Geometry: final body of the model. Coordinates: model frame, mm. A direction names the side the tool comes from. Coordinates: 2 decimals unless noted, no trailing zeros. Loops run counter-clockwise (first coordinate to the right, second up) from the corner with the lowest first, then second, coordinate; pieces in that order, holes last. Notation, with made-up numbers: (48.5, 45.25) - (104.5, 45.25) arc R28 cw to (104.5, 65.25) - close; hole circle Ø10 at (-17, -35.5). An arc over 180 degrees is marked (long way). Answer in a Markdown table with one row per item.
from build123d import *

# Parameters (mm, degrees)
SKETCH1_R           = 8.5
BOSS_EXTRUDE1_DEPTH = 61
SKETCH9_R           = 1.7
CUT_EXTRUDE2_DEPTH  = 6.7
SKETCH10_R          = 1
CUT_EXTRUDE3_DEPTH  = 8.7
CIRPATTERN1_COUNT   = 4
SKETCH11_R          = 1.7
CUT_EXTRUDE4_DEPTH  = 8.7


with BuildPart() as part:
    # Sketch1 → Boss-Extrude1 (new body)
    with BuildSketch(Plane.XY):
        with Locations(Location((0, 0, 0), (0, 0, 180))):
            Circle(SKETCH1_R)
    extrude(amount=BOSS_EXTRUDE1_DEPTH)

    # Sketch7 → Cut-Revolve1 (revolve, cut)
    with BuildSketch(Plane(origin=(0, 0, 0), x_dir=(0, 0, -1), z_dir=(1, 0, 0)), mode=Mode.PRIVATE) as cut_revolve1_sk:
        Polygon((-61, 3), (-5, 3), (-1, 1.5), (0, 1.5), (0, 0), (-61, 0), align=None)
    revolve(cut_revolve1_sk.sketch.rotate(Axis((0, 0, 0), (0, 0, 1)), 90), axis=Axis((0, 0, 0), (0, 0, 1)), mode=Mode.SUBTRACT)

    # Sketch9 → Cut-Extrude2 (cut)
    with BuildSketch(Plane(origin=(8.5, 0, 0), x_dir=(0, 0, -1), z_dir=(1, 0, 0))):
        with Locations((-6.641615966, 0)):
            Circle(SKETCH9_R)
    extrude(amount=-CUT_EXTRUDE2_DEPTH, mode=Mode.SUBTRACT)

    # Sketch10 → Cut-Extrude3 (cut)
    with BuildSketch(Plane(origin=(0, 0, 0), x_dir=(0, 0, -1), z_dir=(1, 0, 0))):
        with Locations(Location((-59, 0, 0), (0, 0, 180))):
            Circle(SKETCH10_R)
    cut_extrude3 = extrude(amount=-CUT_EXTRUDE3_DEPTH, mode=Mode.SUBTRACT)

    # CirPattern1: Cut-Extrude3 ×4 about axis
    cirpattern1_axis = Axis((0, 0, 61), (0, 0, 1))
    for i in range(1, CIRPATTERN1_COUNT):
        add(cut_extrude3.rotate(cirpattern1_axis, i * 360 / CIRPATTERN1_COUNT), mode=Mode.SUBTRACT)

    # Sketch11 → Cut-Extrude4 (cut)
    with BuildSketch(Plane(origin=(0, 8.5, 0), x_dir=(1, 0, 0), z_dir=(0, 1, 0))):
        with Locations(Location((0, -31.611405642, 0), (0, 0, 270))):
            Circle(SKETCH11_R)
    extrude(amount=-CUT_EXTRUDE4_DEPTH, mode=Mode.SUBTRACT)


solid = part.part
(1) Ray query, probe 1 along Z at (x, y) = (6.25, 0); probe 2 along Y at (x, z) = (0, 19.5); probe 3 along Z at (x, y) = (0, -4.65). Return the intervals inside material, ascending.
Verdict:
| item | result |
|---|---|
| probe 1 | z = 0 to 4.94, 8.34 to 58, 60 to 61 |
| probe 2 | y = -8.5 to -3, 3 to 8.5 |
| probe 3 | z = 0 to 58, 60 to 61 |
(2) Cut plane D-D on z = 51. Output: boundary loops of the cut face in (x, y), then the cut area to 3 significant figures.
Verdict:
| item | result |
|---|---|
| outline | circle Ø17 at (0, 0); hole circle Ø6 at (0, 0) |
| area | 199 mm² |
(3) Cut plane B-B on z = 59. Output: boundary loops of the cut face in (x, y), then the cut area to 3 significant figures.
Verdict:
| item | result |
|---|---|
| outline | (-8.44, -1) arc R8.5 ccw to (-1, -8.44) - (-1, -2.83) arc R3 cw to (-2.83, -1) - close; (-8.44, 1) - (-2.83, 1) arc R3 cw to (-1, 2.83) - (-1, 8.44) arc R8.5 ccw to start; (1, -8.44) arc R8.5 ccw to (8.44, -1) - (2.83, -1) arc R3 cw to (1, -2.83) - close; (1, 2.83) arc R3 cw to (2.83, 1) - (8.44, 1) arc R8.5 ccw to (1, 8.44) - close |
| area | 154 mm² |
(4) Cut plane A-A on x = 0. Output: boundary loops of the cut face in (y, z).
Verdict:
| item | result |
|---|---|
| outline | (-8.5, 0) - (-1.5, 0) - (-1.5, 1) - (-3, 5) - (-3, 58) - (-8.5, 58) - close; (-8.5, 60) - (-3, 60) - (-3, 61) - (-8.5, 61) - close; (1.5, 0) - (8.5, 0) - (8.5, 29.91) - (3, 29.91) - (3, 5) - (1.5, 1) - close; (3, 33.31) - (8.5, 33.31) - (8.5, 58) - (3, 58) - close; (3, 60) - (8.5, 60) - (8.5, 61) - (3, 61) - close |
(5) Cut plane C-C on x = 7.25. Output: boundary loops of the cut face in (y, z), then the cut area to 3 significant figures.
Verdict:
| item | result |
|---|---|
| outline | (-4.44, 0) - (4.44, 0) - (4.44, 61) - (-4.44, 61) - close; hole circle Ø3.4 at (0, 6.64); hole circle Ø2 at (0, 59) |
| area | 529 mm² |
(6) First-contact query: pin 1 Ø1 at (y, z) = (-5.5, 16) entering from -X; pin 2 Ø1.8 at (y, z) = (0, 59) entering from -X; pin 3 Ø1.5 at (x, z) = (-6, 46) entering from +Y; pin 4 Ø4 at (x, z) = (2.5, 34) entering from +Y. Flat tips, straight axial feed; report the tip coordinate or a pass-through.
Verdict:
| item | result |
|---|---|
| pin 1 | stops at x = -6.87 |
| pin 2 | passes through |
| pin 3 | stops at y = 6.68 |
| pin 4 | stops at y = 8.49 |
(7) Pull-direction query (X, two-part tool) for faces 6 (the face through (-1.43, -0.45, 0.49)), 7 (the face through (1.107, -8.428, 30.073)), 8 (the face through (-6, 0, 58)); classes: pulls with the +X half, pulls with the -X half, needs draft (parallel to the pull), parting line crosses it, or undercut.
Verdict:
| item | result |
|---|---|
| face 6 | undercut |
| face 7 | parting line crosses it |
| face 8 | needs draft |
(8) Access query for faces 1 (the face through (5.53, 0.07, 8.34)), 2 (the face through (0, -6, 58)), 3 (the face through (6, 0, 58)), 4 (the face through (0.075, 5.528, 29.913)), 5 (the face through (-2.86, -0.9, 32.61)). Directions: +Z, -Z, +X, -X, +Y, -Y. A direction counts if a zero-diameter tool reaches every point of the face in a straight line with its end or side. Return the directions, or none.
Verdict:
| item | result |
|---|---|
| face 1 | +X |
| face 2 | +Y, -Y |
| face 3 | +X, -X |
| face 4 | +Y |
| face 5 | +Z |
